Can you work these out from the model? Positions are in its coordinate system, mm. A direction names the side the tool comes from. Give positions to 0.01 mm unless a question says otherwise; leave off trailing zeros. Order: outer loops, then holes, each group sorted by start corner. A loop starts at its lowest first (then second) coordinate and runs counter-clockwise, first axis right, second up. Notation, with made-up numbers: M 31.25,48.5 L 45.25,48.5 A8 ccw 45.25,59.5 Z; hole C 78.25,4.25 d6. An arc over 180 degrees is marked long. Answer as a JSON object with one key per item and string values.
```python
from build123d import *

# Parameters (mm, degrees)
F0_W     = 40
F0_H     = 40
F0_R     = 1.75
F1_DEPTH = 3
F2_W     = 24
F2_H     = 6
F3_DEPTH = 24
F4_R     = 9
F5_DEPTH = 25
F6_DEPTH = 24
F7_SIZE  = 15
F8_R     = 4


with BuildPart() as f1:
    # F0 (on Top) → F1 (new body)
    with BuildSketch(Plane.XY):
        Rectangle(F0_W, F0_H)
        with Locations((-16.25, -16.25)):
            Circle(F0_R, mode=Mode.SUBTRACT)
        with Locations((16.25, -16.25)):
            Circle(F0_R, mode=Mode.SUBTRACT)
        with Locations((-16.25, 16.25)):
            Circle(F0_R, mode=Mode.SUBTRACT)
        with Locations((16.25, 16.25)):
            Circle(F0_R, mode=Mode.SUBTRACT)
    extrude(amount=F1_DEPTH)

    # F2 (on face) → F3 (join)
    with BuildSketch(Plane.XY.offset(3)):
        with Locations((0, -17)):
            Rectangle(F2_W, F2_H)
    extrude(amount=F3_DEPTH)

    # F4 (on face) → F5 (cut)
    with BuildSketch(Plane(origin=(0, -14, 0), x_dir=(-1, 0, 0), z_dir=(0, 1, 0))):
        with Locations((0, 15)):
            Circle(F4_R)
    extrude(amount=-F5_DEPTH, mode=Mode.SUBTRACT)

    # F6 (add): a face of the model
    f6_faces = [f1.faces().sort_by_distance(p)[0] for p in [
        (20, 0, 1.5),
    ]]
    extrude(f6_faces, amount=F6_DEPTH)

    # F7
    f7_edges = [f1.edges().sort_by_distance(p)[0] for p in [
        (44, 20, 1.5),
        (44, -20, 1.5),
    ]]
    chamfer(f7_edges, length=F7_SIZE)

    # F8
    f8_edges = [f1.edges().sort_by_distance(p)[0] for p in [
        (29, 20, 1.5),
        (44, 5, 1.5),
        (-20, 20, 1.5),
        (-20, -20, 1.5),
        (29, -20, 1.5),
        (44, -5, 1.5),
        (-12, -17, 27),
        (12, -17, 27),
    ]]
    fillet(f8_edges, radius=F8_R)


solid = f1.part
```
1) I need wall thicknesses on L1, parallel to Y at x = -16.25, z = 1.3; L2, parallel to Y at x = 7.5, z = 7.75; L3, parallel to Z at x = -6, y = 11. Which ranges of each line are inside material? Lowest first, please.
Results found:
{"L1": "y = -19.99 to -18, -14.5 to 14.5, 18 to 19.99", "L2": "y = -20 to -14", "L3": "z = 0 to 3"}
2) Thinking about a two-plate mould opening in Y: for faces 1 (the face through (-16.478, -14.515, 1.479)), 2 (the face through (28.854, -19.704, 1.521)), 3 (the face through (-12, -17, 13)), which applies, pulls with the +Y half, pulls with the -Y half, needs draft (parallel to the pull), parting line crosses it, or undercut?
Results found:
{"face 1": "undercut", "face 2": "pulls with the -Y half", "face 3": "needs draft"}
3) I'm going to push flat-ended pins straight in: pin 1 Ø12 at (x, z) = (4, 10) entering from +Y; pin 2 Ø4.5 at (x, y) = (-16.25, -16.25) entering from +Z; pin 3 Ø3 at (y, z) = (-17, 10.5) entering from +X. Where does each tip first touch, or does it pass through?
Results found:
{"pin 1": "stops at y = -14", "pin 2": "stops at z = 3", "pin 3": "stops at x = 12"}
4) I want a section at B-B on x = 0. Write out the boundary of the cut face in (y, z), and give its area (3 significant figures).
Results found:
{"outline": "M -20,0 L 20,0 L 20,3 L -14,3 L -14,6 L -20,6 Z; M -20,24 L -14,24 L -14,27 L -20,27 Z", "area": "156 mm²"}
5) I want a section at D-D on y = 10. Write out the boundary of the cut face in (x, z), and give its area (3 significant figures).
Results found:
{"outline": "M -20,0 L 39,0 L 39,3 L -20,3 Z", "area": "177 mm²"}
6) I want a section at A-A on z = 15. Write out the boundary of the cut face in (x, y), and give its area (3 significant figures).
Results found:
{"outline": "M -12,-20 L -9,-20 L -9,-14 L -12,-14 Z; M 9,-20 L 12,-20 L 12,-14 L 9,-14 Z", "area": "36.0 mm²"}
7) For faces 4 (the face through (37, 12, 1)), 5 (the face through (5, -14, 7)), which set-ups out of +Z, -Z, +X, -X, +Y, -Y let a thin tool reach every point of the face, with its end or its side?
Results found:
{"face 4": "+Z, -Z, +X, +Y", "face 5": "+Z, +X, -X, +Y"}
8) I want a section at C-C on x = 16.25. Write out the boundary of the cut face in (y, z).
Results found:
{"outline": "M -20,0 L -18,0 L -18,3 L -20,3 Z; M -14.5,0 L 14.5,0 L 14.5,3 L -14.5,3 Z; M 18,0 L 20,0 L 20,3 L 18,3 Z"}
